Part model, mm, in its own coordinate system. Face numbers are marked on the shaded views. A direction names the side the tool comes from. Round coordinates to 2 decimals unless told otherwise and drop trailing zeros. Write each loop counter-clockwise with the first axis right and the second up, starting at its lowest first coordinate (ties: lowest second). Pieces come first, ordered by that corner, then holes. Notation, with made-up numbers: M 71.5,70.5 L 116.5,70.5 A21 cw 116.5,90.5 Z; hole C -40,69.25 d6. An arc over 180 degrees is marked long. Answer as a JSON object with one key per item and string values. Group by question number.
1. Drill centre lines: line 1 (X direction, y = 4, z = -2); line 2 (Z direction, x = 6, y = 0.75); line 3 (Y direction, x = 5.75, z = -1.75). Where is each one in solid material? Low to high. Write a range as from..to.
2. Which spindle directions (+Z, -Z, +X, -X, +Y, -Y) get a long thin tool onto all of the face, cutting with end or side? Do the marked faces 1, 2 and 3. Say none if no direction does.
3. Drop a flat-ended pin along its axis: pin 1 (1.8 mm diameter, centred on x = -7, z = 0.5, fed in from -Y). Give the stop position or say it passes through.
4. Two-plate mould, pull along X, no slides. Class the marked faces 4, 5 and 6: +X half, -X half, draft (parallel to the pull), parting line (faces both ways), or undercut.
5. Band-saw the part on A-A, the plane y = 2.75. Write the cut outline in (x, z), plus the area to 3 significant figures.
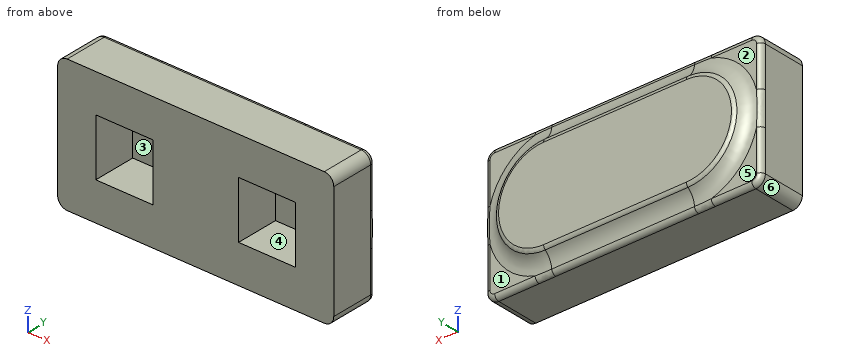
Autodesk Inventor part; units mm, degrees
ref_plane "YZ Plane" through (0, 0, 0) normal (1, 0, 0) x (0, 1, 0)
ref_plane "XZ Plane" through (0, 0, 0) normal (0, 1, 0) x (-1, 0, 0)
ref_plane "XY Plane" through (0, 0, 0) normal (0, 0, 1) x (1, 0, 0)
sketch "Sketch1" plane through (0, 0, 0) normal (0, 1, 0) x (-1, 0, 0)
  line L0 (14.5, 7) -> (-14.5, 7)
  line L1 (-14.5, 7) -> (-14.5, -7)
  line L2 (-14.5, -7) -> (14.5, -7)
  line L3 (14.5, -7) -> (14.5, 7)
  point P0 (0, 0)
  dimension "d0" = 29
  dimension "d1" = 14
  dimension "d2" = 7
  dimension "d3" = 14.5
extrude "Extrusion1" add sketch "Sketch1" along normal blind 5
sketch "Sketch2" plane through (0, 5, 0) normal (0, 1, 0) x (1, 0, 0)
  circle A0 centre (-7.5, 0) radius 5
  circle A1 centre (7.5, 0) radius 5
  line L0 (-14.5, 7) -> (-14.5, -7)
  line L1 (14.5, 7) -> (-14.5, 7)
  line L2 (14.5, -7) -> (14.5, 7)
  line L3 (-7.5, -5) -> (7.5, -5)
  line L4 (-7.5, 5) -> (7.5, 5)
  point P0 (0, 0)
  dimension "d6" = 10
  dimension "d7" = 10
  dimension "d8" = 7
  dimension "d9" = 7
  dimension "d10" = 7
  dimension "d11" = 7
  dimension "d12" = 5
  dimension "d13" = 5
extrude "Extrusion2" add sketch "Sketch2" along normal blind 1
fillet "Fillet1" radius 2 4 edges at (-12.5, 5, 0) (0, 5, -5) (12.5, 5, 0) (0, 5, 5)
fillet "Fillet2" radius 1 4 edges at (14.5, 2.5, 7) (14.5, 2.5, -7) (-14.5, 2.5, -7) (-14.5, 2.5, 7)
fillet "Fillet3" radius 0.5 12 edges at (14.2071, 5, 6.7071) (14.5, 5, 0) (14.2071, 5, -6.7071) (0, 5, -7) (-14.2071, 5, -6.7071) (-14.5, 5, 0) (-14.2071, 5, 6.7071) (0, 5, 7) (-12.5, 6, 0) (0, 6, 5) (12.5, 6, 0) (0, 6, -5)
sketch "Sketch6" plane through (0, 0, 0) normal (0, -1, 0) x (1, 0, 0)
  line L0 (10.5, 3) -> (4.5, 3)
  line L1 (4.5, 3) -> (4.5, -3)
  line L2 (4.5, -3) -> (10.5, -3)
  line L3 (10.5, -3) -> (10.5, 3)
  line L4 (-4.5, 3) -> (-10.5, 3)
  line L5 (-10.5, 3) -> (-10.5, -3)
  line L6 (-10.5, -3) -> (-4.5, -3)
  line L7 (-4.5, -3) -> (-4.5, 3)
  line L8 (-13.5, 7) -> (13.5, 7)
  line L9 (14.5, 6) -> (14.5, -6)
  line L10 (-14.5, -6) -> (-14.5, 6)
  point P0 (0, 0)
  dimension "d43" = 6
  dimension "d44" = 6
  dimension "d45" = 6
  dimension "d46" = 6
  dimension "d47" = 4
  dimension "d48" = 4
  dimension "d49" = 4
  dimension "d50" = 4
extrude "Extrusion7" cut sketch "Sketch6" against normal blind 4.5
properties part number "Keyboard Button"
Worked answers:
{
 "1": {"line 1": "x = -14.5..-10.5, -4.5..4.5, 10.5..14.5", "line 2": "z = -7..-3, 3..7", "line 3": "y = 4.5..6"},
 "2": {"face 1": "-Z, +X, +Y", "face 2": "+Z, -X, +Y", "face 3": "-Y"},
 "3": {"pin 1": "stops at y = 4.5"},
 "4": {"face 4": "undercut", "face 5": "draft", "face 6": "-X half"},
 "5": {"outline": "M -14.5,-6 A1 ccw -13.5,-7 L 13.5,-7 A1 ccw 14.5,-6 L 14.5,6 A1 ccw 13.5,7 L -13.5,7 A1 ccw -14.5,6 Z; hole M -10.5,-3 L -4.5,-3 L -4.5,3 L -10.5,3 Z; hole M 4.5,-3 L 10.5,-3 L 10.5,3 L 4.5,3 Z", "area": "333 mm^2"}
}
